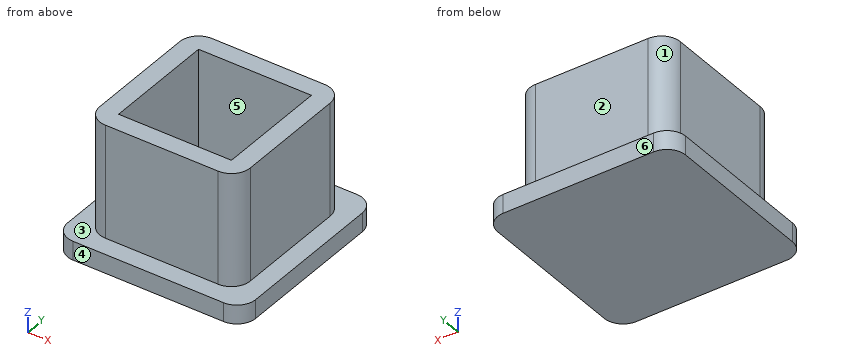
from build123d import *

# Parameters (mm, degrees)
F0_W     = 20
F0_H     = 20
F1_DEPTH = 2
F2_W     = 16
F2_H     = 16
F2_W_2   = 12
F2_H_2   = 12
F3_DEPTH = 12
F4_R     = 2


with BuildPart() as f1:
    # F0 (on Top) → F1 (new body)
    with BuildSketch(Plane.XY):
        Rectangle(F0_W, F0_H)
    extrude(amount=F1_DEPTH)

    # F2 (on face) → F3 (join)
    with BuildSketch(Plane.XY.offset(2)):
        Rectangle(F2_W, F2_H)
        Rectangle(F2_W_2, F2_H_2, mode=Mode.SUBTRACT)
    extrude(amount=F3_DEPTH)

    # F4
    f4_edges = [f1.edges().sort_by_distance(p)[0] for p in [
        (-10, 10, 1),
        (-8, 8, 8),
        (-10, -10, 1),
        (-8, -8, 8),
        (10, 10, 1),
        (8, 8, 8),
        (10, -10, 1),
        (8, -8, 8),
    ]]
    fillet(f4_edges, radius=F4_R)


solid = f1.part
The model under review builds one solid part; all positions refer to its coordinate system, in mm. Face numbers are marked on the shaded views. A direction names the side the tool comes from. Give positions to 0.01 mm unless a question says otherwise; leave off trailing zeros. Write each loop counter-clockwise with the first axis right and the second up, starting at its lowest first coordinate (ties: lowest second). Pieces come first, ordered by that corner, then holes.
1. Wall thickness on L1, parallel to Y at x = 4, z = 12; L2, parallel to Z at x = 0.5, y = -9: over which ranges is each line inside the solid? List them lowest first.
2. Add section D-D, the plane x = 6.75. Write out the cut boundary in (y, z).
3. Add section B-B, the plane x = -4.5. Write out the cut boundary in (y, z), plus the area to 3 significant figures.
4. For P1, Ø3, axis at x = 0, z = 6.5, coming from the -Y side; P2, Ø3.5, axis at y = 0.5, z = 7.5, coming from the -X side; P3, Ø3.5, axis at y = 0.5, z = 10, coming from the +X side, all flat-tipped, find the tip position at first contact; note any pin that passes through.
5. Draft analysis for pull direction Y (two halves, no side actions). For the marked faces 4, 5 and 6, state which applies: +Y half, -Y half, draft (parallel to the pull), parting line (faces both ways), or undercut.
6. Add section A-A, the plane z = 5. Write out the cut boundary in (x, y), plus the area to 3 significant figures.
7. Tool access review of the marked faces 1, 2 and 3: name each direction out of +Z, -Z, +X, -X, +Y, -Y from which nothing blocks a thin tool from reaching the whole face with its end or side.
Worked answers:
1. L1: y = -8 to -6, 6 to 8
1. L2: z = 0 to 2
2. outline: (-10, 0) - (10, 0) - (10, 2) - (7.85, 2) - (7.85, 14) - (-7.85, 14) - (-7.85, 2) - (-10, 2) - close
3. outline: (-10, 0) - (10, 0) - (10, 2) - (8, 2) - (8, 14) - (6, 14) - (6, 2) - (-6, 2) - (-6, 14) - (-8, 14) - (-8, 2) - (-10, 2) - close
3. area: 88.0 mm2
4. P1: stops at y = -8
4. P2: stops at x = -8
4. P3: stops at x = 8
5. face 4: -Y half
5. face 5: undercut
5. face 6: +Y half
6. outline: (-8, -6) arc R2 ccw to (-6, -8) - (6, -8) arc R2 ccw to (8, -6) - (8, 6) arc R2 ccw to (6, 8) - (-6, 8) arc R2 ccw to (-8, 6) - close; hole (-6, -6) - (6, -6) - (6, 6) - (-6, 6) - close
6. area: 109 mm2
7. face 1: +Z, -X, +Y
7. face 2: +Z, +X, -X, +Y
7. face 3: +Z
